Read the model definition and answer for the solid it produces. Units are mm, in the model's axes. A direction names the side the tool comes from. Coordinates: 2 decimals unless noted, no trailing zeros. Loops run counter-clockwise (first coordinate to the right, second up) from the corner with the lowest first, then second, coordinate; pieces in that order, holes last. Notation, with made-up numbers: M 58.25,83.25 L 98.25,83.25 A28 ccw 98.25,118.25 Z; hole C 7,-29 d11. An arc over 180 degrees is marked long. Put each result on its own line as item: value.
from build123d import *

# Parameters (mm, degrees)
CAP_PLATE_26X20X2_START           = -12.4
CAP_PLATE_26X20X2_PROFILE_W       = 26
CAP_PLATE_26X20X2_PROFILE_H       = 20
CAP_PLATE_26X20X2_PROFILE_R       = 6.6
CAP_PLATE_26X20X2_PROFILE_R_2     = 1.1
CAP_PLATE_26X20X2_DEPTH           = 2
BEARING_RETENTION_LIP_START       = -10.41
BEARING_RETENTION_LIP_PROFILE_R   = 8
BEARING_RETENTION_LIP_PROFILE_R_2 = 6.6
BEARING_RETENTION_LIP_DEPTH       = 2.21


with BuildPart() as part:
    # Cap_plate_26x20x2_Profile → Cap_plate_26x20x2 (new body)
    with BuildSketch(Plane.XY.offset(CAP_PLATE_26X20X2_START)):
        with Locations((12.5, 0)):
            Rectangle(CAP_PLATE_26X20X2_PROFILE_W, CAP_PLATE_26X20X2_PROFILE_H)
        with Locations((12.5, 0)):
            Circle(CAP_PLATE_26X20X2_PROFILE_R, mode=Mode.SUBTRACT)
        with Locations((1.8, 0)):
            Circle(CAP_PLATE_26X20X2_PROFILE_R_2, mode=Mode.SUBTRACT)
        with Locations((23.2, 0)):
            Circle(CAP_PLATE_26X20X2_PROFILE_R_2, mode=Mode.SUBTRACT)
    extrude(amount=CAP_PLATE_26X20X2_DEPTH)

    # Bearing_retention_lip_Profile → Bearing_retention_lip (add)
    with BuildSketch(Plane.XY.offset(BEARING_RETENTION_LIP_START)):
        with Locations(Location((12.5, 0, 0), (0, 0, 180))):
            Circle(BEARING_RETENTION_LIP_PROFILE_R)
        with Locations((12.5, 0)):
            Circle(BEARING_RETENTION_LIP_PROFILE_R_2, mode=Mode.SUBTRACT)
    extrude(amount=BEARING_RETENTION_LIP_DEPTH)


solid = part.part
1) Given pin 1 Ø10 at (x, y) = (6.5, 0.5) entering from +Z; pin 2 Ø1 at (y, z) = (4, -9.5) entering from -X; pin 3 Ø1 at (x, z) = (16.5, -9) entering from +Y, each flat-ended and moving along its own axis, determine where each tip first touches the part or whether it passes through.
Answer list:
pin 1: stops at z = -8.2
pin 2: stops at x = 5.31
pin 3: stops at y = 7.19
2) Find section A-A, the plane x = 23.2. Write down the section's boundary in (y, z), plus the area to 3 significant figures.
Answer list:
outline: M -10,-12.4 L -1.1,-12.4 L -1.1,-10.4 L -10,-10.4 Z; M 1.1,-12.4 L 10,-12.4 L 10,-10.4 L 1.1,-10.4 Z
area: 35.6 mm^2
3) Determine the mould class of faces 1 (the flat face through (12, 7, -12.4)), 2 (the cylindrical face through (5.906, 0.29, -10.329)), 3 (the cylindrical face through (1.66, 1.09, -11.41)), 4 (the flat face through (12, -10, -11)) for opening direction Y: released by +Y, released by -Y, zero draft, split by the parting line, or undercut.
Answer list:
face 1: zero draft
face 2: undercut
face 3: undercut
face 4: released by -Y
4) Find section C-C, the plane y = 0. Write down the section's boundary in (x, z), plus the area to 3 significant figures.
Answer list:
outline: M -0.5,-12.4 L 0.7,-12.4 L 0.7,-10.4 L -0.5,-10.4 Z; M 2.9,-12.4 L 5.9,-12.4 L 5.9,-8.2 L 4.5,-8.2 L 4.5,-10.4 L 2.9,-10.4 Z; M 19.1,-12.4 L 22.1,-12.4 L 22.1,-10.4 L 20.5,-10.4 L 20.5,-8.2 L 19.1,-8.2 Z; M 24.3,-12.4 L 25.5,-12.4 L 25.5,-10.4 L 24.3,-10.4 Z
area: 23.0 mm^2
5) Find section B-B, the plane z = -12. Write down the section's boundary in (x, y).
Answer list:
outline: M -0.5,-10 L 25.5,-10 L 25.5,10 L -0.5,10 Z; hole C 1.8,0 d2.2; hole C 12.5,0 d13.2; hole C 23.2,0 d2.2
6) Straight lines are drawn through the part: line 1 (Y direction, x = 12.5, z = -9.5); line 2 (Y direction, x = 23.2, z = -11.15); line 3 (Z direction, x = 24.25, y = -1). For each, find the intervals that lie inside material, in ascending order. Write a range as [from, to].
Answer list:
line 1: y = [-8, -6.6], [6.6, 8]
line 2: y = [-10, -1.1], [1.1, 10]
line 3: z = [-12.4, -10.4]
7) Find section D-D, the plane z = -8.6. Write down the section's boundary in (x, y), plus the area to 3 significant figures.
Answer list:
outline: C 12.5,0 d16; hole C 12.5,0 d13.2
area: 64.2 mm^2
8) Which of the six approach directions +Z, -Z, +X, -X, +Y, -Y give full straight-line access (tool end or side, diameter ignored) to faces 5 (the flat face through (4, 0, -10.4)), 6 (the cylindrical face through (22.33, -0.67, -11.41))?
Answer list:
face 5: +Z
face 6: +Z, -Z
